Answer from the drawing. Dimensions are ordinates in mm from the lowest x, y and z of the part. Round coordinates to 2 decimals unless told otherwise and drop trailing zeros. Loops run counter-clockwise (first coordinate to the right, second up) from the corner with the lowest first, then second, coordinate; pieces in that order, holes last.
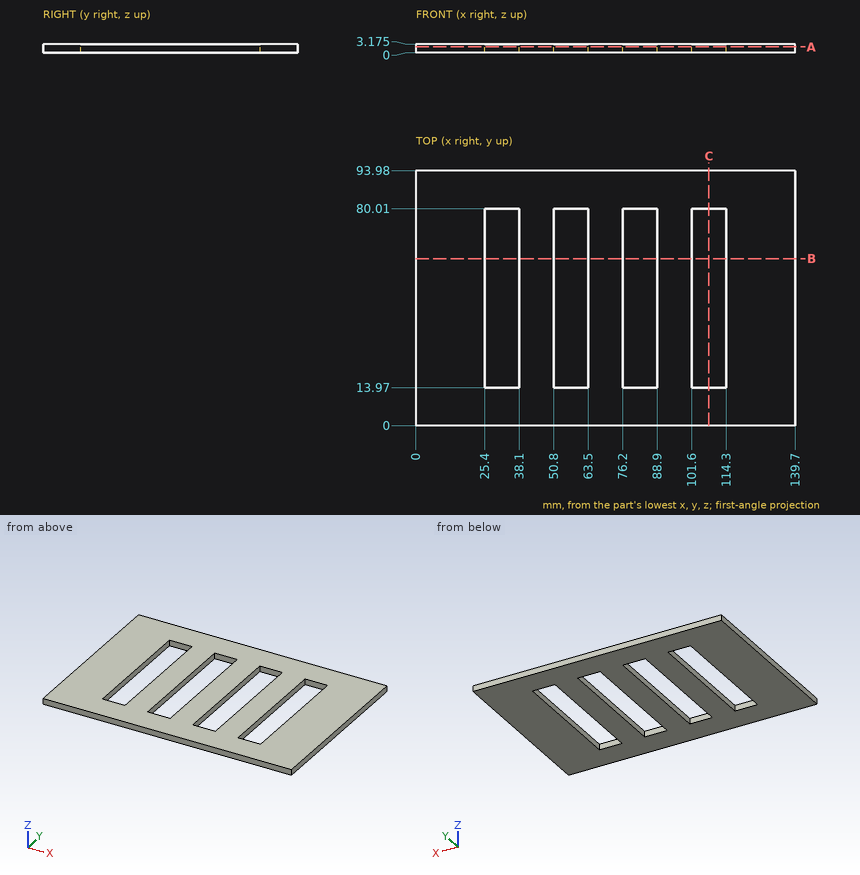
1. Consider probe 1 along X at (y, z) = (62, 0.8); probe 2 along Y at (x, z) = (88.5, 2.65). Determine where each line is inside the solid, lowest interval first.
Answer key:
probe 1: x = 0 to 25.4, 38.1 to 50.8, 63.5 to 76.2, 88.9 to 101.6, 114.3 to 139.7
probe 2: y = 0 to 13.97, 80.01 to 93.98
2. Given pin 1 (1 mm diameter, centred on y = 29.5, z = 0.5, fed in from -X), flat-ended and moving along its own axis, determine where the tip first touches the part or whether it passes through.
Answer key:
pin 1: stops at x = 0
3. Find section A-A (z = 2.1). Write down the section's boundary in (x, y).
Answer key:
outline: (0, 0) - (139.7, 0) - (139.7, 93.98) - (0, 93.98) - close; hole (25.4, 13.97) - (38.1, 13.97) - (38.1, 80.01) - (25.4, 80.01) - close; hole (50.8, 13.97) - (63.5, 13.97) - (63.5, 80.01) - (50.8, 80.01) - close; hole (76.2, 13.97) - (88.9, 13.97) - (88.9, 80.01) - (76.2, 80.01) - close; hole (101.6, 13.97) - (114.3, 13.97) - (114.3, 80.01) - (101.6, 80.01) - close
4. Find section B-B (y = 61.5). Write down the section's boundary in (x, z) (3 decimals), then the cut area to 3 significant figures.
Answer key:
outline: (0, 0) - (25.4, 0) - (25.4, 3.175) - (0, 3.175) - close; (38.1, 0) - (50.8, 0) - (50.8, 3.175) - (38.1, 3.175) - close; (63.5, 0) - (76.2, 0) - (76.2, 3.175) - (63.5, 3.175) - close; (88.9, 0) - (101.6, 0) - (101.6, 3.175) - (88.9, 3.175) - close; (114.3, 0) - (139.7, 0) - (139.7, 3.175) - (114.3, 3.175) - close
area: 282 mm2
5. Find section C-C (x = 108). Write down the section's boundary in (y, z) (3 decimals).
Answer key:
outline: (0, 0) - (13.97, 0) - (13.97, 3.175) - (0, 3.175) - close; (80.01, 0) - (93.98, 0) - (93.98, 3.175) - (80.01, 3.175) - close
